Geometry check sheet. Reference: the model listing, model coordinates, mm. Face numbers are marked on the shaded views. Coordinates: 2 decimals unless noted, no trailing zeros. Order: outer loops, then holes, each group sorted by start corner. A loop starts at its lowest first (then second) coordinate and runs counter-clockwise, first axis right, second up. Notation, with made-up numbers: (18.25, 81) -> (24.25, 81) arc R15 cw to (24.25, 107) -> close; hole circle Ø3 at (33.25, 2.25). An arc over 180 degrees is marked (long way). Answer as CSV lines item,"result". Start each with the question number.
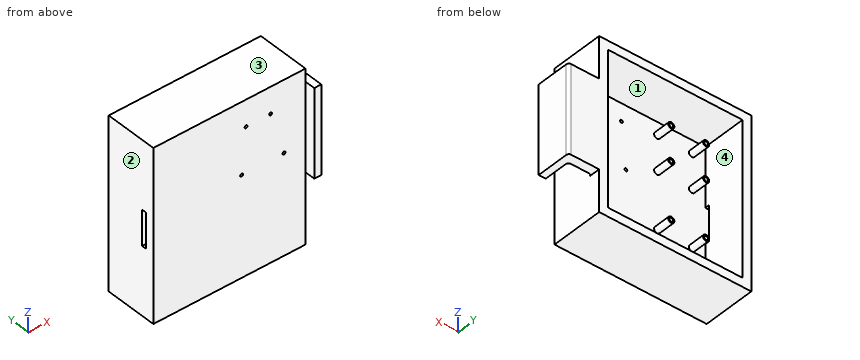
from build123d import *

# Parameters (mm, degrees)
CROQUIS1_W              = 173.1
CROQUIS1_H              = 194.252873564
SALIENTE_EXTRUIR1_DEPTH = 60
VACIADO1_T              = -10
CROQUIS2_R              = 3.5
CROQUIS2_R_2            = 2.165
SALIENTE_EXTRUIR2_DEPTH = 19
CROQUIS3_R              = 1.59
CROQUIS3_R_2            = 1.5875
CORTAR_EXTRUIR1_DEPTH   = 19
CROQUIS5_W              = 40
CROQUIS5_H              = 5
CORTAR_EXTRUIR2_DEPTH   = 19
CROQUIS6_W              = 26.9
CROQUIS6_H              = 100
SALIENTE_EXTRUIR3_DEPTH = 10
CROQUIS7_W              = 8
CROQUIS7_H              = 100
SALIENTE_EXTRUIR4_DEPTH = 40
REDONDEO1_R             = 3
REDONDEO2_R             = 3


with BuildPart() as part:
    # Croquis1 → Saliente-Extruir1 (new body)
    with BuildSketch(Plane(origin=(0, 0, 0), x_dir=(1, 0, 0), z_dir=(0, 1, 0))):
        with Locations((-113.45, 0)):
            Rectangle(CROQUIS1_W, CROQUIS1_H)
    extrude(amount=SALIENTE_EXTRUIR1_DEPTH)

    # Vaciado1
    vaciado1_openings = [part.faces().sort_by_distance(p)[0] for p in [
        (-113.45, 60, 0),
    ]]
    offset(amount=VACIADO1_T, openings=vaciado1_openings, kind=Kind.INTERSECTION)

    # Croquis2 → Saliente-Extruir2 (add)
    # profile 1 of 4: a face of its own
    with BuildSketch(Plane(origin=(0, 10, 0), x_dir=(1, 0, 0), z_dir=(0, 1, 0))):
        with Locations(Location((-135.185, 32.311436782, 0), (0, 0, 270))):
            Circle(CROQUIS2_R)
        with Locations(Location((-135.185, 32.311436782, 0), (0, 0, 270))):
            Circle(CROQUIS2_R_2, mode=Mode.SUBTRACT)
    # profile 2 of 4: a face of its own
    with BuildSketch(Plane(origin=(0, 10, 0), x_dir=(1, 0, 0), z_dir=(0, 1, 0))):
        with Locations(Location((-174.835, 32.311436782, 0), (0, 0, 270))):
            Circle(CROQUIS2_R)
        with Locations(Location((-174.835, 32.311436782, 0), (0, 0, 270))):
            Circle(CROQUIS2_R_2, mode=Mode.SUBTRACT)
    # profile 3 of 4: a face of its own
    with BuildSketch(Plane(origin=(0, 10, 0), x_dir=(1, 0, 0), z_dir=(0, 1, 0))):
        with Locations(Location((-174.835, 71.961436782, 0), (0, 0, 270))):
            Circle(CROQUIS2_R)
        with Locations(Location((-174.835, 71.961436782, 0), (0, 0, 270))):
            Circle(CROQUIS2_R_2, mode=Mode.SUBTRACT)
    # profile 4 of 4: a face of its own
    with BuildSketch(Plane(origin=(0, 10, 0), x_dir=(1, 0, 0), z_dir=(0, 1, 0))):
        with Locations(Location((-135.185, 71.961436782, 0), (0, 0, 270))):
            Circle(CROQUIS2_R)
        with Locations(Location((-135.185, 71.961436782, 0), (0, 0, 270))):
            Circle(CROQUIS2_R_2, mode=Mode.SUBTRACT)
    saliente_extruir2 = extrude(amount=SALIENTE_EXTRUIR2_DEPTH)

    # Simetría1: Saliente-Extruir2 across plane
    add(saliente_extruir2.mirror(Plane.XY))

    # Croquis3 → Cortar-Extruir1 (cut)
    # profile 1 of 5: a face of its own
    with BuildSketch(Plane(origin=(0, 10, 0), x_dir=(1, 0, 0), z_dir=(0, 1, 0))):
        with Locations(Location((-99.618504427, -16.326436782, 0), (0, 0, 270))):
            Circle(CROQUIS3_R)
    # profile 2 of 5: a face of its own
    with BuildSketch(Plane(origin=(0, 10, 0), x_dir=(1, 0, 0), z_dir=(0, 1, 0))):
        with Locations(Location((-51.358504427, -16.326436782, 0), (0, 0, 270))):
            Circle(CROQUIS3_R)
    # profile 3 of 5: a face of its own
    with BuildSketch(Plane(origin=(0, 10, 0), x_dir=(1, 0, 0), z_dir=(0, 1, 0))):
        with Locations(Location((-94.538504427, -67.126436782, 0), (0, 0, 270))):
            Circle(CROQUIS3_R)
    # profile 4 of 5: a face of its own
    with BuildSketch(Plane(origin=(0, 10, 0), x_dir=(1, 0, 0), z_dir=(0, 1, 0))):
        with Locations(Location((-66.598504427, -67.126436782, 0), (0, 0, 270))):
            Circle(CROQUIS3_R)
    # profile 5 of 5: a face of its own
    with BuildSketch(Plane(origin=(0, 10, 0), x_dir=(1, 0, 0), z_dir=(0, 1, 0))):
        Polygon((12.20327424, 3.574424869), (9.66327424, 1.034424869), (-3.29072576, 1.034424869), (-3.29072576, -65.005575131), (50.04927424, -65.005575131), (50.04927424, 1.034424869), (47.50927424, 1.034424869), (44.96927424, 3.574424869), align=None)
        with Locations((14.48927424, 1.034424869)):
            Circle(CROQUIS3_R_2, mode=Mode.SUBTRACT)
        with Locations((42.42927424, 1.034424869)):
            Circle(CROQUIS3_R_2, mode=Mode.SUBTRACT)
        with Locations((47.50927424, -51.035575131)):
            Circle(CROQUIS3_R_2, mode=Mode.SUBTRACT)
        with Locations((-0.75072576, -49.765575131)):
            Circle(CROQUIS3_R_2, mode=Mode.SUBTRACT)
    extrude(amount=-CORTAR_EXTRUIR1_DEPTH, mode=Mode.SUBTRACT)

    # Croquis5 → Cortar-Extruir2 (cut)
    with BuildSketch(Plane(origin=(-190, 0, 0), x_dir=(0, 0, -1), z_dir=(1, 0, 0))):
        with Locations((0, 12.5)):
            Rectangle(CROQUIS5_W, CROQUIS5_H)
    extrude(amount=-CORTAR_EXTRUIR2_DEPTH, mode=Mode.SUBTRACT)

    # Croquis6 → Saliente-Extruir3 (add)
    with BuildSketch(Plane(origin=(0, 60, 0), x_dir=(1, 0, 0), z_dir=(0, 1, 0))):
        with Locations((-13.45, 0)):
            Rectangle(CROQUIS6_W, CROQUIS6_H)
    extrude(amount=-SALIENTE_EXTRUIR3_DEPTH)

    # Croquis7 → Saliente-Extruir4 (add)
    with BuildSketch(Plane(origin=(0, 60, 0), x_dir=(1, 0, 0), z_dir=(0, 1, 0))):
        with Locations((4, 0)):
            Rectangle(CROQUIS7_W, CROQUIS7_H)
    extrude(amount=-SALIENTE_EXTRUIR4_DEPTH)

    # Redondeo1
    redondeo1_edges = [part.edges().sort_by_distance(p)[0] for p in [
        (-26.9, 50, 0),
        (0, 50, 0),
    ]]
    fillet(redondeo1_edges, radius=REDONDEO1_R)

    # Redondeo2
    redondeo2_edges = [part.edges().sort_by_distance(p)[0] for p in [
        (8, 60, 0),
    ]]
    fillet(redondeo2_edges, radius=REDONDEO2_R)


solid = part.part
Q1. Sectioned sample at A-A, the plane y = 32. Record the cut outline in (x, z).
Q2. Sectioned sample at B-B, the plane x = -147. Record the cut outline in (y, z), then the cut area to 3 significant figures.
Q3. Sectioned sample at C-C, the plane z = 52.5. Record the cut outline in (x, y), then the cut area to 3 significant figures.
Q4. Release check for a two-part mould opening along X. For the marked faces 1, 2, 3 and 4 record: released by +X, released by -X, zero draft, split by the parting line, or undercut.
Q5. Sectioned sample at D-D, the plane y = 4. Record the cut outline in (x, z), then the cut area to 3 significant figures.
Q6. Thickness scan on L1, parallel to X at y = 32.5, z = 3; L2, parallel to Z at x = -48, y = 33; L3, parallel to X at y = 57.5, z = -30. Record the ranges inside material, lowest first.
Q7. Go/stop test with flat-tipped pins: pin 1 Ø5 at (x, z) = (-174, 72.5) entering from +Y; pin 2 Ø1 at (y, z) = (46.5, -67.5) entering from +X; pin 3 Ø1.5 at (x, z) = (-91.5, -38) entering from +Y. Record where each tip stops, or that it passes through.
Geometry results:
1,outline,"(-200, -97.13) -> (-26.9, -97.13) -> (-26.9, 97.13) -> (-200, 97.13) -> close; (0, -50) -> (8, -50) -> (8, 50) -> (0, 50) -> close; hole (-190, -87.13) -> (-36.9, -87.13) -> (-36.9, 87.13) -> (-190, 87.13) -> close"
2,outline,"(0, -97.13) -> (60, -97.13) -> (60, -87.13) -> (10, -87.13) -> (10, 87.13) -> (60, 87.13) -> (60, 97.13) -> (0, 97.13) -> close"
2,area,"2,940 mm^2"
3,outline,"(-200, 0) -> (-26.9, 0) -> (-26.9, 60) -> (-36.9, 60) -> (-36.9, 10) -> (-190, 10) -> (-190, 60) -> (-200, 60) -> close"
3,area,"2,730 mm^2"
4,face 1,"undercut"
4,face 2,"released by -X"
4,face 3,"zero draft"
4,face 4,"undercut"
5,outline,"(-200, -97.13) -> (-26.9, -97.13) -> (-26.9, 97.13) -> (-200, 97.13) -> close; hole circle Ø3.18 at (-99.62, 16.33); hole circle Ø3.18 at (-94.54, 67.13); hole circle Ø3.18 at (-66.6, 67.13); hole circle Ø3.18 at (-51.36, 16.33)"
5,area,"33,600 mm^2"
6,L1,"x = -200 to -190, -36.9 to -26.9, 0 to 8"
6,L2,"z = -97.13 to -87.13, 87.13 to 97.13"
6,L3,"x = -200 to -190, -36.9 to 7.96"
7,pin 1,"stops at y = 29"
7,pin 2,"stops at x = -26.9"
7,pin 3,"stops at y = 10"
